Could you check a few things on this model? Use its own coordinates, in mm. A direction names the side the tool comes from. Round coordinates to 2 decimals unless told otherwise and drop trailing zeros. Write each loop counter-clockwise with the first axis right and the second up, starting at its lowest first coordinate (ties: lowest second). Pieces come first, ordered by that corner, then holes. Notation, with made-up numbers: (75, 84) -> (123, 84) arc R27 ccw to (123, 109) -> close; hole circle Ø4 at (23.25, 57). An arc over 180 degrees is marked (long way). Answer in a Markdown table with one row per item.
from build123d import *

# Parameters (mm, degrees)
SKETCH_1_R        = 45
SKETCH_1_R_2      = 30
EXTRUDE_5_DEPTH   = 40
SKETCH_1_R_3      = 20
SKETCH_1_R_4      = 10
EXTRUDE_5_2_DEPTH = 40
EXTRUDE_START     = 35
SKETCH_1_7_R      = 45
SKETCH_1_7_R_2    = 20
EXTRUDE_6_DEPTH   = 8


with BuildPart() as part:
    # Sketch 1 → Extrude 5 (new, symmetric)
    with BuildSketch(Plane.XY):
        Circle(SKETCH_1_R)
        Circle(SKETCH_1_R_2, mode=Mode.SUBTRACT)
    extrude(amount=EXTRUDE_5_DEPTH, both=True)



with BuildPart() as body_2:
    # Sketch 1 → Extrude 5 2 (new, symmetric)
    with BuildSketch(Plane.XY):
        with Locations((106, 0)):
            Circle(SKETCH_1_R_3)
        with Locations((106, 0)):
            Circle(SKETCH_1_R_4, mode=Mode.SUBTRACT)
    extrude(amount=EXTRUDE_5_2_DEPTH, both=True)


with BuildPart() as part_1:
    add(part.part)

    add(body_2.part)  # Extrude 6 merges body 2
    # Sketch 1_7 → Extrude 6 (add)
    with BuildSketch(Plane.XY.offset(EXTRUDE_START)):
        with BuildLine():
            Line((113.134433962, 26.558423373), (14.268867925, 53.116846745))
            ThreePointArc((14.268867925, 53.116846745), (-55, 0), (14.268867925, -53.116846745))
            Line((14.268867925, -53.116846745), (113.134433962, -26.558423373))
            ThreePointArc((113.134433962, -26.558423373), (133.5, 0), (113.134433962, 26.558423373))
        make_face()
        Circle(SKETCH_1_7_R, mode=Mode.SUBTRACT)
        with Locations((106, 0)):
            Circle(SKETCH_1_7_R_2, mode=Mode.SUBTRACT)
    extrude_6 = extrude(amount=-EXTRUDE_6_DEPTH)

    # Mirror 2: Extrude 6 across plane
    add(extrude_6.mirror(Plane.XY))


solid = part_1.part
1) Thinking about a two-plate mould opening in Z: for faces 1 (the face through (86.02, 0.88, 0.38)), 2 (the face through (29, -9, -40)), 3 (the face through (46, 4, -27)), 4 (the face through (64.394, 39.652, -31.056)), which applies, +Z half, -Z half, draft (parallel to the pull), parting line (faces both ways), or undercut?
Findings:
| item | result |
|---|---|
| face 1 | undercut |
| face 2 | -Z half |
| face 3 | undercut |
| face 4 | draft |
2) Please list where these lines run through material, in increasing order: line 1 (Z direction, x = -39, y = -28); line 2 (Y direction, x = 0, z = 5); line 3 (Y direction, x = -9.5, z = 19.5).
Findings:
| item | result |
|---|---|
| line 1 | z = -35 to -27, 27 to 35 |
| line 2 | y = -45 to -30, 30 to 45 |
| line 3 | y = -43.99 to -28.46, 28.46 to 43.99 |
3) Imagine slicing it at A-A, the plane x = 0. Please give me the cut outline in (y, z).
Findings:
| item | result |
|---|---|
| outline | (-55, -35) -> (-45, -35) -> (-45, -40) -> (-30, -40) -> (-30, 40) -> (-45, 40) -> (-45, 35) -> (-55, 35) -> (-55, 27) -> (-45, 27) -> (-45, -27) -> (-55, -27) -> close; (30, -40) -> (45, -40) -> (45, -35) -> (55, -35) -> (55, -27) -> (45, -27) -> (45, 27) -> (55, 27) -> (55, 35) -> (45, 35) -> (45, 40) -> (30, 40) -> close |
4) Imagine slicing it at C-C, the plane z = 7. Please give me the cut outline in (x, y).
Findings:
| item | result |
|---|---|
| outline | circle Ø90 at (0, 0); circle Ø40 at (106, 0); hole circle Ø60 at (0, 0); hole circle Ø20 at (106, 0) |
5) For pin 1 (1 mm diameter, centred on y = 26.5, z = -9.5, fed in from +X); pin 2 (10 mm diameter, centred on y = 8.5, z = -13, fed in from -X); pin 3 (8 mm diameter, centred on x = 9.5, z = 16.5, fed in from +Y), each with a flat end and sliding along its axis, tell me the tip position at first contact or that it passes through.
Findings:
| item | result |
|---|---|
| pin 1 | stops at x = 36.73 |
| pin 2 | stops at x = -44.86 |
| pin 3 | stops at y = 44.66 |
6) For faces 5 (the face through (46, 4, 27)), 6 (the face through (86.02, 0.88, -37.47)), 7 (the face through (97, 5, 40)), 8 (the face through (46, 4, 35)), which set-ups out of +Z, -Z, +X, -X, +Y, -Y let a thin tool reach every point of the face, with its end or its side?
Findings:
| item | result |
|---|---|
| face 5 | none |
| face 6 | -Z |
| face 7 | +Z, +X, -X, +Y, -Y |
| face 8 | +Z |
7) Imagine slicing it at D-D, the plane x = 106. Please give me the cut outline in (y, z).
Findings:
| item | result |
|---|---|
| outline | (-28.47, -35) -> (-20, -35) -> (-20, -40) -> (-10, -40) -> (-10, 40) -> (-20, 40) -> (-20, 35) -> (-28.47, 35) -> (-28.47, 27) -> (-20, 27) -> (-20, -27) -> (-28.47, -27) -> close; (10, -40) -> (20, -40) -> (20, -35) -> (28.47, -35) -> (28.47, -27) -> (20, -27) -> (20, 27) -> (28.47, 27) -> (28.47, 35) -> (20, 35) -> (20, 40) -> (10, 40) -> close |
8) Imagine slicing it at B-B, the plane y = 0. Count the separate pieces of the cut face and the enclosed holes in it, plus the area to 3 significant figures.
Findings:
| item | result |
|---|---|
| separate pieces | 3 |
| enclosed holes | 1 |
| area | 4,940 mm^2 |
